Geometry: final body of the model. Coordinates: model frame, mm. A direction names the side the tool comes from. Coordinates: 2 decimals unless noted, no trailing zeros. Loops run counter-clockwise (first coordinate to the right, second up) from the corner with the lowest first, then second, coordinate; pieces in that order, holes last. Notation, with made-up numbers: (67, 82) - (84, 82) arc R29 cw to (84, 121) - close; hole circle Ø7 at (-4.75, -8.75). An arc over 180 degrees is marked (long way). Return JSON: item names as keys, results as strings.
Autodesk Inventor part; units mm, degrees
ref_plane "YZ Plane" through (0, 0, 0) normal (1, 0, 0) x (0, 1, 0)
ref_plane "XZ Plane" through (0, 0, 0) normal (0, 1, 0) x (-1, 0, 0)
ref_plane "XY Plane" through (0, 0, 0) normal (0, 0, 1) x (1, 0, 0)
sketch "Sketch1" plane through (0, 0, 0) normal (0, 0, 1) x (1, 0, 0)
  line L0 (0, 0) -> (25.4, 0)
  line L1 (25.4, 0) -> (25.4, 25.4)
  line L2 (25.4, 25.4) -> (0, 25.4)
  line L3 (0, 25.4) -> (0, 0)
  circle A0 centre (12.7, 12.7) radius 3.5687
  dimension "d0" = 25.4
  dimension "d1" = 25.4
  dimension "d2" = 7.1374
extrude "Extrusion1" add sketch "Sketch1" along normal blind 4.7752
sketch "Sketch2" plane through (0, 0, 4.7752) normal (0, 0, 1) x (1, 0, 0)
  line L0 (25.4, 25.4) -> (0, 25.4)
  line L1 (0, 0) -> (4.7752, 0)
  line L2 (4.7752, 0) -> (4.7752, 25.4)
  line L3 (4.7752, 25.4) -> (0, 25.4)
  line L4 (0, 25.4) -> (0, 0)
  dimension "d5" = 4.7752
extrude "Extrusion2" add sketch "Sketch2" against normal blind 25.4
sketch "Sketch3" plane through (4.7752, 0, 0) normal (1, 0, 0) x (0, 0, -1)
  line L0 (20.6248, 25.4) -> (20.6248, 0)
  circle A0 centre (7.9248, 12.7) radius 3.5687
  point P0 (0, 0)
  dimension "d9" = 7.1374
extrude "Extrusion3" cut sketch "Sketch3" against normal up to next
fillet "Fillet1" radius 4.7625 1 edges at (4.7752, 12.7, -20.6248)
fillet "Fillet2" radius 4.7625 1 edges at (25.4, 12.7, 0)
properties part number "8020_CornerBracket"
Item 1: Reachability of faces 1 (the face through (9, 10, 0)), 2 (the face through (6.9, 0, 0.4)) from +Z, -Z, +X, -X, +Y, -Y: full face, straight path, thin tool, end or side. Return the list, or none.
Worked out:
{"face 1": "-Z, +X, +Y, -Y", "face 2": "+Z, -Z, +X, -X, -Y"}
Item 2: Mould query, pull axis X, two halves, no side actions, for faces 3 (the face through (3.42, 12.88, -19.19)), 4 (the face through (0, 10, -11)), 5 (the face through (9.135, 12.543, 2.354)). Classes: +X half, -X half, draft (parallel to the pull), parting line (faces both ways), or undercut.
Worked out:
{"face 3": "+X half", "face 4": "-X half", "face 5": "undercut"}
Item 3: Ray query, probe 1 along Y at (x, z) = (12.7, 2.4); probe 2 along X at (y, z) = (5.5, -11.25). Return the intervals inside material, ascending. Write a range as from..to.
Worked out:
{"probe 1": "0..9.13, 16.27..25.4", "probe 2": "0..4.78"}
Item 4: Section query A-A, the plane y = 12.7. Count the separate pieces of the cut face and the enclosed holes in it, and give its area (3 significant figures).
Worked out:
{"separate pieces": "3", "enclosed holes": "0", "area": "142 mm^2"}
Item 5: First-contact query: pin 1 Ø6 at (x, y) = (21.5, 19.5) entering from -Z; pin 2 Ø2 at (y, z) = (21, -15) entering from +X. Flat tips, straight axial feed; report the tip coordinate or a pass-through.
Worked out:
{"pin 1": "z = 0", "pin 2": "x = 4.78"}
Item 6: Section query B-B, the plane x = 12.7. Return loops of the section in (y, z).
Worked out:
{"outline": "(0, 0) - (9.13, 0) - (9.13, 4.78) - (0, 4.78) - close; (16.27, 0) - (25.4, 0) - (25.4, 4.78) - (16.27, 4.78) - close"}
Item 7: Section query D-D, the plane x = 8.5. Return loops of the section in (y, z).
Worked out:
{"outline": "(0, 0) - (25.4, 0) - (25.4, 4.78) - (0, 4.78) - close"}
